For this review, take the finished solid that the model builds, in its own axes (mm). A direction names the side the tool comes from. Give positions to 0.01 mm unless a question says otherwise; leave off trailing zeros. Write each loop counter-clockwise with the first axis right and the second up, starting at its lowest first coordinate (ties: lowest second). Pieces come first, ordered by that corner, then holes. Notation, with made-up numbers: M -6,-17 L 1,-17 A28 ccw 1,5 Z; hole C 46.25,-13 d2. An arc over 180 degrees is marked long. Use one line per item in the form item = value. Start each with the question number.
Q1. Tool access review of faces 1 (the flat face through (-13, -76.722, 38)), 2 (the cylindrical face through (-37.922, 3.05, 18.265)): name each direction out of +Z, -Z, +X, -X, +Y, -Y from which nothing blocks a thin tool from reaching the whole face with its end or side.
Q2. Clearance check with flat-ended pins moving along their axes: pin 1 Ø0.6 at (x, y) = (13, 0.5) entering from +Z; pin 2 Ø2 at (x, y) = (15, 0.5) entering from -Z; pin 3 Ø12 at (y, z) = (45.5, 16.5) entering from -X. State where each tip first meets the part, or that it passes through.
Q3. Consider section C-C on x = -41. Write out the cut boundary in (y, z).
Q4. For probe 1 along X at (y, z) = (21.5, 52); probe 2 along Y at (x, z) = (-33, 31); probe 3 along Z at (x, y) = (-37, -7.5), list the stretches that pass through material, from the lowest coordinate up. Write a range as [from, to].
Q5. Consider section A-A on y = -34.5. Write out the cut boundary in (x, z), and give its area (3 significant figures).
Q6. Consider section B-B on z = 61. Write out the cut boundary in (x, y).
```python
from build123d import *

# Parameters (mm, degrees)
F0_W     = 83.83190725
F0_H     = 76.6697376966
F1_DEPTH = 25.4
F3_DEPTH = 68.58
F6_DEPTH = 25.4
F7_R     = 14.0713154884
F8_DEPTH = 25.4


with BuildPart() as f1:
    # F0 (on Right) → F1 (new body)
    with BuildSketch(Plane.YZ):
        with Locations((33.7740029208, 38.3348688483)):
            Rectangle(F0_W, F0_H)
    extrude(amount=-F1_DEPTH)

    # F3 (add): a face of the model
    f3_faces = [f1.faces().sort_by_distance(p)[0] for p in [
        (-12.7, -8.1419507042, 38.3348688483),
    ]]
    extrude(f3_faces, amount=F3_DEPTH)

    # F5 (on face) → F6 (join)
    with BuildSketch(Plane.YZ):
        Polygon((2.735585974, 46.5573131723), (0.9166808596, 46.7870943248), (-0.9166808596, 46.7870943248), (-2.735585974, 46.5573131723), (-4.5113492634, 46.1013746532), (-6.2159658801, 45.4264691904), (-7.8225530015, 44.5432404463), (-9.3057737891, 43.4656174656), (-10.6422369651, 42.2105950066), (-11.8108657068, 40.7979655232), (-12.7932300408, 39.2500070262), (-13.5738374948, 37.5911317457), (-14.1403774229, 35.847501136), (-14.4839151519, 34.0466132933), (-14.5990328868, 32.2168692946), (-14.4839151519, 30.387125296), (-14.1403774229, 28.5862374533), (-13.5738374948, 26.8426068436), (-12.7932300408, 25.1837315631), (-11.8108657068, 23.6357730661), (-10.6422369651, 22.2231435827), (-9.3057737891, 20.9681211237), (-7.8225530015, 19.890498143), (-6.2159658801, 19.0072693989), (-4.5113492634, 18.3323639361), (-2.735585974, 17.876425417), (-0.9166808596, 17.6466442645), (0.9166808596, 17.6466442645), (2.735585974, 17.876425417), (4.5113492634, 18.3323639361), (6.2159658801, 19.0072693989), (7.8225530015, 19.890498143), (9.3057737891, 20.9681211237), (10.6422369651, 22.2231435827), (11.8108657068, 23.6357730661), (12.7932300408, 25.1837315631), (13.5738374948, 26.8426068436), (14.1403774229, 28.5862374533), (14.4839151519, 30.387125296), (14.5990328868, 32.2168692946), (14.4839151519, 34.0466132933), (14.1403774229, 35.847501136), (13.5738374948, 37.5911317457), (12.7932300408, 39.2500070262), (11.8108657068, 40.7979655232), (10.6422369651, 42.2105950066), (9.3057737891, 43.4656174656), (7.8225530015, 44.5432404463), (6.2159658801, 45.4264691904), (4.5113492634, 46.1013746532), align=None)
    extrude(amount=F6_DEPTH)

    # F7 (on face) → F8 (join)
    with BuildSketch(Plane(origin=(-25.4, 0, 0), x_dir=(0, -1, 0), z_dir=(-1, 0, 0))):
        with Locations((0, 32.0016257465)):
            Circle(F7_R)
    extrude(amount=F8_DEPTH)


solid = f1.part
```
Working result:
q1.face_1 = +Z, -Z, +X, -X, -Y
q1.face_2 = -X
q2.pin_1 = 46.79
q2.pin_2 = 17.65
q2.pin_3 = -25.4
q3.outline = C 0,32 d28.14
q4.probe_1 = [-25.4, 0]
q4.probe_2 = [-14.04, 14.04]
q4.probe_3 = [20.1, 43.91]
q5.outline = M -25.4,0 L 0,0 L 0,76.67 L -25.4,76.67 Z
q5.area = 1,950 mm²
q6.outline = M -25.4,-76.72 L 0,-76.72 L 0,75.69 L -25.4,75.69 Z
